```python
from build123d import *

# Parameters (mm, degrees)
BOSS_EXTRUDE1_DEPTH = 12.5
FILLET1_R           = 1.5
SKETCH3_R           = 1.45
SKETCH3_R_2         = 3.75
CUT_EXTRUDE1_DEPTH  = 60.036005962
SKETCH5_R           = 1.6
CUT_EXTRUDE2_DEPTH  = 59.182901268
CUT_EXTRUDE3_DEPTH  = 59.182901268
FILLET2_R           = 6.4


with BuildPart() as part:
    # Sketch1 → Boss-Extrude1 (new, symmetric)
    with BuildSketch(Plane(origin=(0, 0, 0), x_dir=(0, 0, -1), z_dir=(1, 0, 0))):
        Polygon((0, 25), (0, 0), (50, 0), (50, -2), (-2, -2), (-2, 25), align=None)
    extrude(amount=BOSS_EXTRUDE1_DEPTH, both=True)

    # Fillet1
    fillet1_edges = [part.edges().sort_by_distance(p)[0] for p in [
        (0, -2, 2),
    ]]
    fillet(fillet1_edges, radius=FILLET1_R)

    # Sketch3 → Cut-Extrude1 (cut, through all)
    with BuildSketch(Plane.XY.offset(2)):
        with BuildLine():
            ThreePointArc((-12.5, 12.5), (-8.838834765, 21.338834765), (0, 25))
            Line((0, 25), (-12.5, 25))
            Line((-12.5, 25), (-12.5, 12.5))
        make_face()
        with BuildLine():
            ThreePointArc((0, 25), (8.838834765, 21.338834765), (12.5, 12.5))
            Line((12.5, 12.5), (12.5, 25))
            Line((12.5, 25), (0, 25))
        make_face()
        with Locations((0, 21)):
            Circle(SKETCH3_R)
        with Locations((0, 12.5)):
            Circle(SKETCH3_R_2)
        with Locations((-8.5, 12.5)):
            Circle(SKETCH3_R)
        with Locations((0, 4)):
            Circle(SKETCH3_R)
        with Locations((8.5, 12.5)):
            Circle(SKETCH3_R)
    extrude(amount=-CUT_EXTRUDE1_DEPTH, mode=Mode.SUBTRACT)

    # Sketch5 → Cut-Extrude2 (cut, through all)
    with BuildSketch(Plane.XZ.offset(2)):
        with Locations(Location((0, -42.8, 0), (0, 0, 270))):
            Circle(SKETCH5_R)
        with Locations(Location((0, -36.4, 0), (0, 0, 270))):
            Circle(SKETCH5_R)
        with Locations(Location((0, -30, 0), (0, 0, 270))):
            Circle(SKETCH5_R)
        with Locations(Location((0, -23.6, 0), (0, 0, 270))):
            Circle(SKETCH5_R)
        with Locations(Location((0, -17.2, 0), (0, 0, 270))):
            Circle(SKETCH5_R)
        with Locations(Location((0, -10.8, 0), (0, 0, 270))):
            Circle(SKETCH5_R)
        with Locations(Location((0, -4.4, 0), (0, 0, 270))):
            Circle(SKETCH5_R)
    extrude(amount=-CUT_EXTRUDE2_DEPTH, mode=Mode.SUBTRACT)

    # Sketch6 → Cut-Extrude3 (cut, through all)
    with BuildSketch(Plane.XZ.offset(2)):
        with BuildLine():
            Line((12.5, -40.95), (12.5, -37.55))
            Line((12.5, -37.55), (10.8, -37.55))
            ThreePointArc((10.8, -37.55), (9.1, -39.25), (10.8, -40.95))
            Line((10.8, -40.95), (12.5, -40.95))
        make_face()
        with BuildLine():
            Line((10.8, -34.6), (12.5, -34.6))
            Line((12.5, -34.6), (12.5, -31.2))
            Line((12.5, -31.2), (10.8, -31.2))
            ThreePointArc((10.8, -31.2), (9.1, -32.9), (10.8, -34.6))
        make_face()
        with BuildLine():
            Line((12.5, -5.8), (10.8, -5.8))
            ThreePointArc((10.8, -5.8), (9.1, -7.5), (10.8, -9.2))
            Line((10.8, -9.2), (12.5, -9.2))
            Line((12.5, -9.2), (12.5, -5.8))
        make_face()
        with BuildLine():
            Line((10.8, -28.25), (12.5, -28.25))
            Line((12.5, -28.25), (12.5, -24.85))
            Line((12.5, -24.85), (10.8, -24.85))
            ThreePointArc((10.8, -24.85), (9.1, -26.55), (10.8, -28.25))
        make_face()
        with BuildLine():
            Line((12.5, -12.15), (10.8, -12.15))
            ThreePointArc((10.8, -12.15), (9.1, -13.85), (10.8, -15.55))
            Line((10.8, -15.55), (12.5, -15.55))
            Line((12.5, -15.55), (12.5, -12.15))
        make_face()
        with BuildLine():
            Line((10.8, -21.9), (12.5, -21.9))
            Line((12.5, -21.9), (12.5, -18.5))
            Line((12.5, -18.5), (10.8, -18.5))
            ThreePointArc((10.8, -18.5), (9.1, -20.2), (10.8, -21.9))
        make_face()
    cut_extrude3 = extrude(amount=-CUT_EXTRUDE3_DEPTH, mode=Mode.SUBTRACT)

    # Mirror1: Cut-Extrude3 across plane
    add(cut_extrude3.mirror(Plane(origin=(0, 0, 0), x_dir=(0, 0, 1), z_dir=(1, 0, 0))), mode=Mode.SUBTRACT)

    # Fillet2
    fillet2_edges = [part.edges().sort_by_distance(p)[0] for p in [
        (12.5, -1, -50),
        (-12.5, -1, -50),
    ]]
    fillet(fillet2_edges, radius=FILLET2_R)


solid = part.part
```
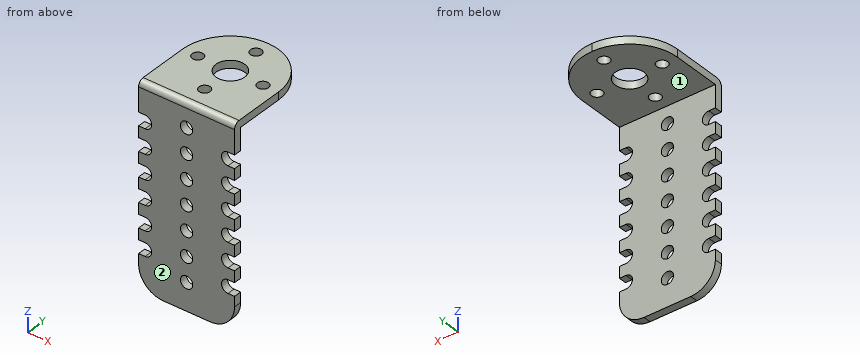
Source: CAD feature listing. Evaluate the final solid. Frame: model axes, mm. Face numbers are marked on the shaded views. A direction names the side the tool comes from. Coordinates: 2 decimals unless noted, no trailing zeros. Order: outer loops, then holes, each group sorted by start corner. A loop starts at its lowest first (then second) coordinate and runs counter-clockwise, first axis right, second up. Notation, with made-up numbers: (81.5, -7.5) - (140.5, -7.5) arc R18 ccw to (140.5, 6.5) - close; hole circle Ø9 at (16.25, -33.5). An arc over 180 degrees is marked (long way). One line per item, written item: value.
1) Cut plane B-B on z = -10.8. Output: boundary loops of the cut face in (x, y), plus the area to 3 significant figures.
Computed values:
outline: (-12.5, -2) - (-1.6, -2) - (-1.6, 0) - (-12.5, 0) - close; (1.6, -2) - (12.5, -2) - (12.5, 0) - (1.6, 0) - close
area: 43.6 mm^2
2) Cut plane A-A on y = 4. Output: boundary loops of the cut face in (x, z).
Computed values:
outline: (-12.5, 0) - (-1.45, 0) - (-1.45, 2) - (-12.5, 2) - close; (1.45, 0) - (12.5, 0) - (12.5, 2) - (1.45, 2) - close
3) Cut plane D-D on z = -40. Output: boundary loops of the cut face in (x, y).
Computed values:
outline: (-9.27, -2) - (9.27, -2) - (9.27, 0) - (-9.27, 0) - close
4) Contact query for flat-ended pins moving along their axis: pin 1 (1 mm diameter, centred on x = -6, y = 14, fed in from -Z); pin 2 (8 mm diameter, centred on x = -7.5, z = -15, fed in from +Y); pin 3 (3 mm diameter, centred on x = 0, z = -42.8, fed in from +Y); pin 4 (1.9 mm diameter, centred on x = 11.5, y = -1, fed in from -Z). Output: stop coordinate, or through.
Computed values:
pin 1: stops at z = 0
pin 2: stops at y = 0
pin 3: passes through
pin 4: stops at z = -48.2
5) Ray query, line 1 (X direction, y = -1.35, z = -10.8); line 2 (Y direction, x = -0.5, z = -1.5); line 3 (Z direction, x = 8.75, y = 20.75). Return the intervals inside material, ascending. Write a range as [from, to].
Computed values:
line 1: x = [-12.5, -1.6], [1.6, 12.5]
line 2: y = [-2, 0]
line 3: z = [0, 2]
6) Cut plane C-C on x = -0.75. State how many separate pieces and enclosed holes the cut face has, plus the area to 3 significant figures.
Computed values:
separate pieces: 11
enclosed holes: 0
area: 89.3 mm^2
7) Reachability of the marked faces 1 and 2 from +Z, -Z, +X, -X, +Y, -Y: full face, straight path, thin tool, end or side. Return the list, or none.
Computed values:
face 1: -Z, +X, -X, +Y
face 2: +Z, -Z, +X, -X, -Y
